```python
from build123d import *

# Parameters (mm, degrees)
SKETCH2_W  = 19.05
SKETCH2_H  = 3.4036
SLOT_DEPTH = 4.9022


with BuildPart() as part:
    # BodySke → BaseBody (revolve)
    with BuildSketch(Plane.XY):
        with BuildLine():
            Line((2.552216058, 9.525), (46.99, 9.525))
            Line((46.99, 9.525), (50.8, 5.715))
            Line((50.8, 5.715), (47.366081562, 0))
            Line((47.366081562, 0), (0, 0))
            ThreePointArc((0, 0), (0.649113009, 4.930502809), (2.552216058, 9.525))
        make_face()
    revolve(axis=Axis((-12.7, 0, 0), (1, 0, 0)))

    # Sketch2 → Slot (cut)
    with BuildSketch(Plane(origin=(0, 0, 0), x_dir=(0, 0, -1), z_dir=(1, 0, 0))):
        Rectangle(SKETCH2_W, SKETCH2_H)
    extrude(amount=SLOT_DEPTH, mode=Mode.SUBTRACT)


solid = part.part
```
Source: CAD feature listing. Evaluate the final solid. Frame: model axes, mm. A direction names the side the tool comes from. Coordinates: 2 decimals unless noted, no trailing zeros. Loops run counter-clockwise (first coordinate to the right, second up) from the corner with the lowest first, then second, coordinate; pieces in that order, holes last. Notation, with made-up numbers: M 0,66 L 55,66 A16 cw 55,92 Z; hole C 51,18.5 d8. An arc over 180 degrees is marked long. Use a Markdown table: item, result. Add a question column.
Q1. First-contact query: pin 1 (4 mm diameter, centred on x = 43, z = -3.5, fed in from +Y); pin 2 (1 mm diameter, centred on y = -2, z = 5, fed in from -X); pin 3 (4 mm diameter, centred on y = -1, z = 2, fed in from +X). Flat tips, straight axial feed; report the tip coordinate or a pass-through.
Q2. Section query A-A, the plane x = 12. Return loops of the section in (y, z) (3 decimals), and give its area (3 significant figures).
Q3. Material intervals for L1, parallel to X at y = -4.75, z = -7.5; L2, parallel to Y at x = 36, z = -1.5; L3, parallel to Y at x = 38, z = -3.5, sorted ascending.
Q4. Access query for faces 1 (the flat face through (3, 1.702, 0)), 2 (the cylindrical face through (25.082, -7.559, -5.796)). Directions: +Z, -Z, +X, -X, +Y, -Y. A direction counts if a zero-diameter tool reaches every point of the face in a straight line with its end or side. Return the directions, or none.
Q5. Draft query along Y for faces 3 (the flat face through (4.902, 0, 0)), 4 (the conical face through (50.615, -1.279, -5.76)), 5 (the conical face through (47.914, -0.198, -0.891)). Return one class per face: pulls with the +Y half, pulls with the -Y half, needs draft (parallel to the pull), parting line crosses it, or undercut.
Result:
| question | item | result |
|---|---|---|
| 1 | pin 1 | stops at y = 9.41 |
| 1 | pin 2 | stops at x = 0.64 |
| 1 | pin 3 | stops at x = 49.91 |
| 2 | outline | C 0,0 d19.05 |
| 2 | area | 285 mm2 |
| 3 | L1 | x = 2.2 to 47.64 |
| 3 | L2 | y = -9.41 to 9.41 |
| 3 | L3 | y = -8.86 to 8.86 |
| 4 | face 1 | +Z, -Z, -X |
| 4 | face 2 | +X, -X |
| 5 | face 3 | undercut |
| 5 | face 4 | parting line crosses it |
| 5 | face 5 | undercut |
